Design review of the part shown in the three views and the two pictorial views. Dimensions are in mm from the part's minimum x, y and z. A direction names the side the tool comes from. Coordinates: 2 decimals unless noted, no trailing zeros. Loops run counter-clockwise (first coordinate to the right, second up) from the corner with the lowest first, then second, coordinate; pieces in that order, holes last. Notation, with made-up numbers: (67, 25) -> (125, 25) arc R33 cw to (125, 58) -> close; hole circle Ø6 at (3, 86). An arc over 180 degrees is marked (long way). Use CSV: the item, a comma, the result in double quotes.
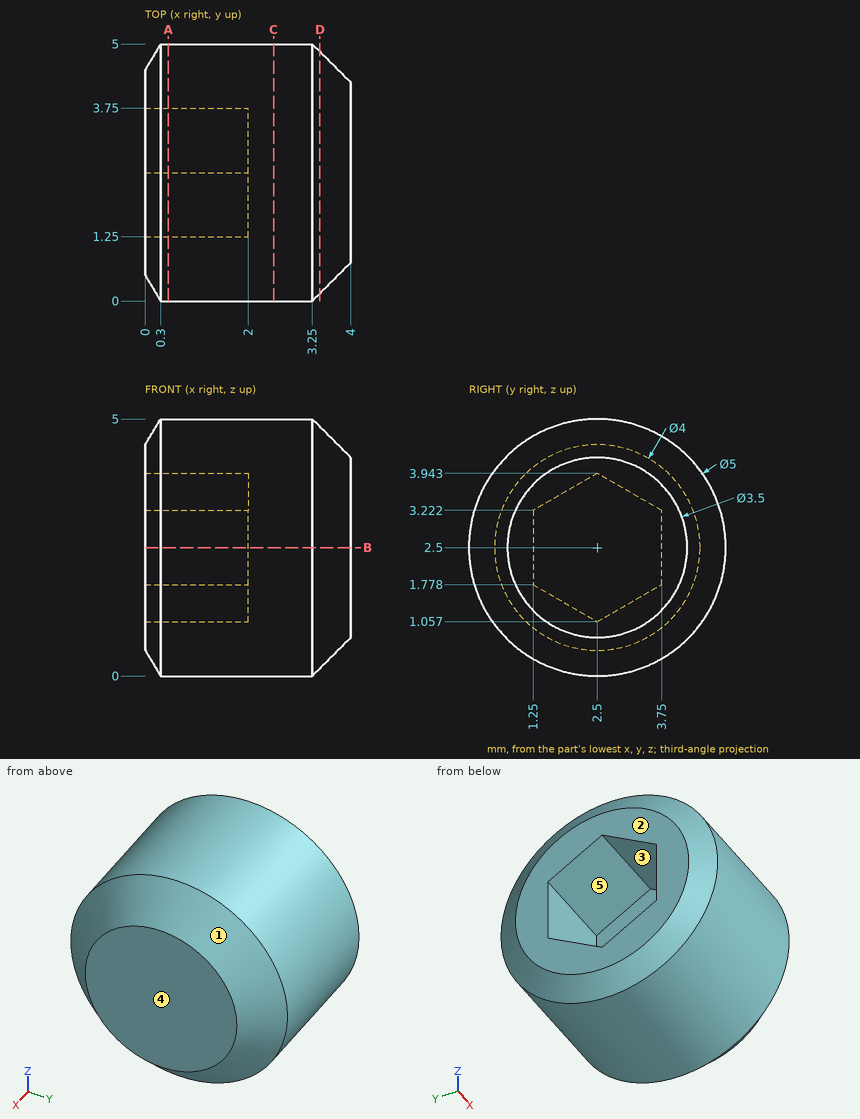
Item 1: Add section A-A (x = 0.45). Give the boundary of the cut face in (y, z).
Checked values:
outline,"circle Ø5 at (2.5, 2.5); hole (1.25, 1.78) -> (2.5, 1.06) -> (3.75, 1.78) -> (3.75, 3.22) -> (2.5, 3.94) -> (1.25, 3.22) -> close"
Item 2: Add section B-B (z = 2.5). Give the boundary of the cut face in (x, y).
Checked values:
outline,"(0, 0.5) -> (0.3, 0) -> (3.25, 0) -> (4, 0.75) -> (4, 4.25) -> (3.25, 5) -> (0.3, 5) -> (0, 4.5) -> (0, 3.75) -> (2, 3.75) -> (2, 1.25) -> (0, 1.25) -> close"
Item 3: Machinability: for the marked faces 4 and 5, which of the approach directions +Z, -Z, +X, -X, +Y, -Y give a long, thin tool a straight path to every point of the face, cutting with its end or side? Answer none if there is none.
Checked values:
face 4,"+Z, -Z, +X, +Y, -Y"
face 5,"-X"
Item 4: Clearance check with flat-ended pins moving along their axes: pin 1 (1.5 mm diameter, centred on x = 2, z = 3, fed in from -Y); pin 2 (0.7 mm diameter, centred on x = 1, z = 2, fed in from +Y). State where each tip first meets the part, or that it passes through.
Checked values:
pin 1,"y = 0"
pin 2,"y = 5"
Item 5: Add section C-C (x = 2.5). Give the boundary of the cut face in (y, z), then the cut area to 3 significant figures.
Checked values:
outline,"circle Ø5 at (2.5, 2.5)"
area,"19.6 mm^2"
Item 6: Draft analysis for pull direction Z (two halves, no side actions). For the marked faces 1, 2 and 3, state which applies: pulls with the +Z half, pulls with the -Z half, needs draft (parallel to the pull), parting line crosses it, or undercut.
Checked values:
face 1,"parting line crosses it"
face 2,"needs draft"
face 3,"undercut"
Item 7: Add section D-D (x = 3.4). Give the boundary of the cut face in (y, z).
Checked values:
outline,"circle Ø4.7 at (2.5, 2.5)"
Item 8: To check wall thickness, follow line 1 along X through (y, z) = (3.1, 3.3); line 2 along Z through (x, y) = (1.1, 2.9); line 3 along Y through (x, z) = (1.5, 0.5). State the ranges of each line that lie inside material, in increasing order.
Checked values:
line 1,"2 to 4"
line 2,"0.03 to 1.29, 3.71 to 4.97"
line 3,"1 to 4"
